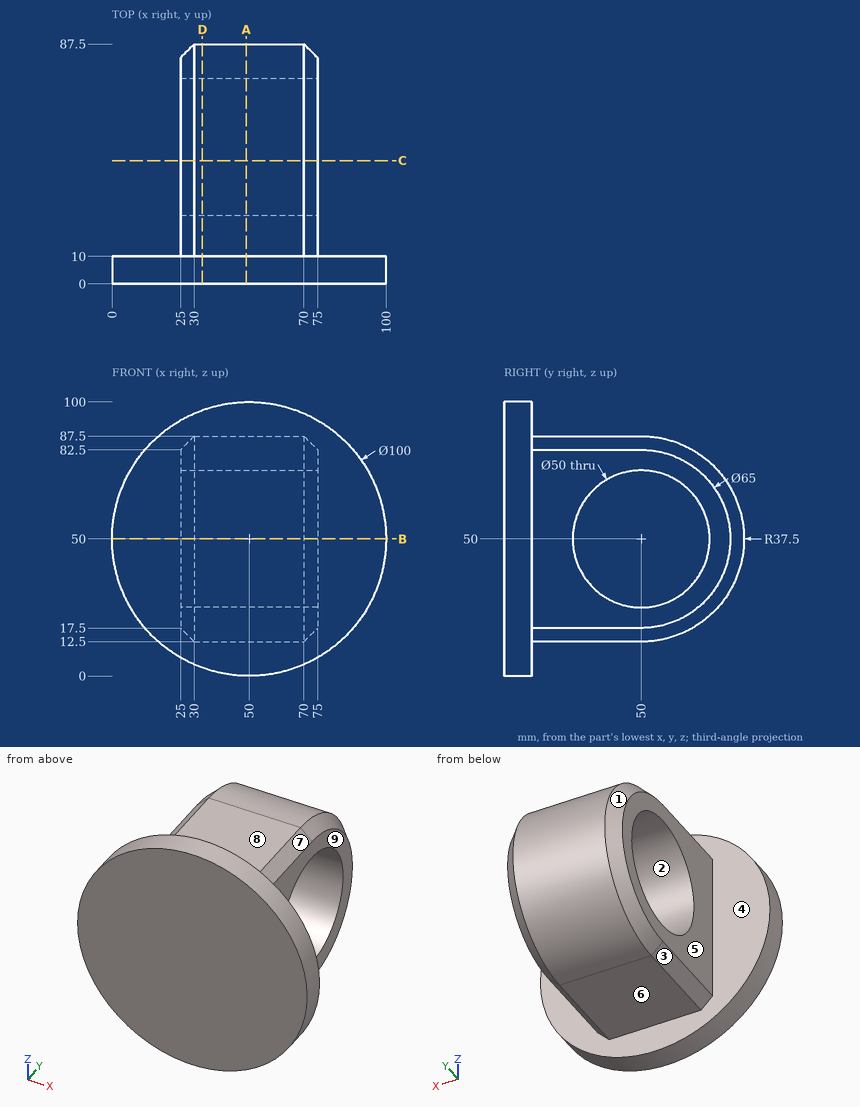
The figure shows three views and two pictorial views of one solid part (mm, origin at its lowest corner). Answer the questions. A direction names the side the tool comes from. Give positions to 0.01 mm unless a question says otherwise; leave off trailing zeros. Write each loop counter-clockwise with the first axis right and the second up, starting at its lowest first coordinate (ties: lowest second). Pieces come first, ordered by that corner, then holes.
Q1. The part is cut by section B-B on z = 50. Give the vertices of the cut face in (x, y), and give its area (3 significant figures).
Answer:
outline: (0, 0) - (100, 0) - (100, 10) - (75, 10) - (75, 25) - (25, 25) - (25, 10) - (0, 10) - close; (25, 75) - (75, 75) - (75, 82.5) - (70, 87.5) - (30, 87.5) - (25, 82.5) - close
area: 2,350 mm2
Q2. Straight lines are drawn through the part: L1, parallel to Y at x = 54, z = 50; L2, parallel to Y at x = 39, z = 27; L3, parallel to Z at x = 55, y = 65. For each, find the intervals that lie inside material, in ascending order.
Answer:
L1: y = 0 to 25, 75 to 87.5
L2: y = 0 to 40.2, 59.8 to 79.62
L3: z = 15.63 to 30, 70 to 84.37
Q3. A tool of negligible diameter and unlimited length cuts with its end or side. For the marked faces 5, 6, 7, 8 and 9, from which of +Z, -Z, +X, -X, +Y, -Y can it reach the whole face along a straight path? Write none if from no direction.
Answer:
face 5: +Z, -Z, -X, +Y
face 6: -Z, +X, -X, +Y
face 7: +Z, +X, +Y
face 8: +Z, +X, -X, +Y
face 9: +Z, -Z, +X, +Y
Q4. For a pull along Z with two mould halves and no side action, classify the marked faces 1, 2, 3 and 4 as released by +Z, released by -Z, zero draft, split by the parting line, or undercut.
Answer:
face 1: split by the parting line
face 2: undercut
face 3: released by -Z
face 4: zero draft
Q5. The part is cut by section C-C on y = 45. Give the vertices of the cut face in (x, z), and give its area (3 significant figures).
Answer:
outline: (25, 17.5) - (30, 12.5) - (70, 12.5) - (75, 17.5) - (75, 25.51) - (25, 25.51) - close; (25, 74.49) - (75, 74.49) - (75, 82.5) - (70, 87.5) - (30, 87.5) - (25, 82.5) - close
area: 1,250 mm2
Q6. Given pin 1 (2 mm diameter, centred on x = 43, z = 28, fed in from +Y); pin 2 (8 mm diameter, centred on x = 49.5, z = 13.5, fed in from +Y); pin 3 (4 mm diameter, centred on x = 56, y = 23, fed in from +Z), each flat-ended and moving along its own axis, determine where each tip first touches the part or whether it passes through.
Answer:
pin 1: stops at y = 81.07
pin 2: stops at y = 68.71
pin 3: stops at z = 87.5
Q7. The part is cut by section D-D on x = 33. Give the vertices of the cut face in (y, z), and give its area (3 significant figures).
Answer:
outline: (0, 2.98) - (10, 2.98) - (10, 12.5) - (50, 12.5) arc R37.5 ccw to (50, 87.5) - (10, 87.5) - (10, 97.02) - (0, 97.02) - close; hole circle Ø50 at (50, 50)
area: 4,190 mm2
Q8. The part is cut by section A-A on x = 49. Give the vertices of the cut face in (y, z), and give its area (3 significant figures).
Answer:
outline: (0, 0.01) - (10, 0.01) - (10, 12.5) - (50, 12.5) arc R37.5 ccw to (50, 87.5) - (10, 87.5) - (10, 99.99) - (0, 99.99) - close; hole circle Ø50 at (50, 50)
area: 4,250 mm2
